Autodesk Inventor part; units mm, degrees
ref_plane "YZ Plane" through (0, 0, 0) normal (1, 0, 0) x (0, 1, 0)
ref_plane "XZ Plane" through (0, 0, 0) normal (0, 1, 0) x (-1, 0, 0)
ref_plane "XY Plane" through (0, 0, 0) normal (0, 0, 1) x (1, 0, 0)
sketch "스케치1" plane through (0, 0, 0) normal (1, 0, 0) x (0, 1, 0)
  line L0 (0, 0) -> (6, 0)
  line L1 (6, 0) -> (6, 15)
  line L2 (6, 15) -> (0, 15)
  line L3 (0, 15) -> (0, 0)
  line L4 (0, 15) -> (8, 15)
  line L5 (8, 15) -> (8, 40)
  line L6 (8, 40) -> (0, 40)
  line L7 (0, 40) -> (0, 15)
  line L8 (0, 40) -> (17, 40)
  line L9 (17, 40) -> (17, 55)
  line L10 (17, 55) -> (0, 55)
  line L11 (0, 55) -> (0, 40)
  line L12 (0, 55) -> (8, 55)
  line L13 (8, 55) -> (8, 80)
  line L14 (8, 80) -> (0, 80)
  line L15 (0, 80) -> (0, 55)
  line L16 (0, 80) -> (6, 80)
  line L17 (6, 80) -> (6, 120)
  line L18 (6, 120) -> (0, 120)
  line L19 (0, 120) -> (0, 80)
  dimension "d0" = 12
  dimension "d1" = 16
  dimension "d2" = 34
  dimension "d3" = 16
  dimension "d4" = 15
  dimension "d5" = 25
  dimension "d6" = 15
  dimension "d7" = 25
  dimension "d9" = 40
  dimension "d10" = 12
revolve "회전1" add sketch "스케치1" angle 360 about axis through (0, 0, 40) along (0, 0, -1)
sketch "스케치2" plane through (0, 0, 55) normal (0, 0, 1) x (1, 0, 0)
  circle A0 centre (0, 0) radius 8
  circle A1 centre (-4.5, 0) radius 12.5
  circle A2 centre (0, 0) radius 17
  point P0 (0, 0)
  dimension "d11" = 25
extrude "돌출1" cut sketch "스케치2" against normal up to next contours A2
sketch "스케치3" plane through (0, 0, 0) normal (0, 0, -1) x (-1, 0, 0)
  circle A0 centre (0, 0) radius 2
  dimension "d14" = 4
hole "구멍1" at (0, 0, 0) direction (0, 0, 1) diameter 3.242 depth 11.8 tip angle 118
sketch "스케치4" plane through (0, 0, 0) normal (1, 0, 0) x (0, 1, 0)
  line L0 (8, 78.2679) -> (8, 80)
  line L1 (8, 80) -> (7, 80)
  line L2 (7, 80) -> (8, 78.2679)
  line L3 (8, 80) -> (8, 55)
  line L4 (-8, 80) -> (8, 80)
  line L5 (0, -24) -> (0, 144)
  point P0 (0, 0)
  dimension "d22" = 30
  dimension "d23" = 1
revolve "회전2" cut sketch "스케치4" angle 360 about axis through (0, 0, -10) along (0, 0, 1)
fillet "모깎기1" radius 4 1 edges at (0, -8, 78.2679)
fillet "모깎기2" radius 1 1 edges at (0, -7, 80)
sketch "스케치5" plane through (0, 0, 0) normal (1, 0, 0) x (0, 1, 0)
  circle A0 centre (8.6, 98) radius 8
  line L0 (6, 120) -> (6, 80)
  point P0 (0, 0)
  dimension "d27" = 16
  dimension "d29" = 5.4
  dimension "d30" = 18
extrude "돌출2" cut sketch "스케치5" along normal mid plane 3
sketch "스케치6" plane through (0, 0, 0) normal (1, 0, 0) x (0, 1, 0)
  line L0 (-4.5, 105) -> (-6, 105)
  line L1 (-6, 105) -> (-6, 103.5)
  line L2 (-6, 103.5) -> (-4.5, 105)
  line L3 (-6, 120) -> (-6, 80)
  point P0 (0, 0)
  dimension "d33" = 1.5
  dimension "d34" = 45
  dimension "d35" = 25
revolve "회전3" cut sketch "스케치6" angle 360 about axis through (0, -4.5, 105) along (0, -1, 0)
chamfer "모따기1" distance 1 angle 45 3 edges at (0, -6, 120) (0, -8, 15) (0, -6, 0)
properties part number "3강"
For this review, take the finished solid that the model builds, in its own axes (mm). A direction names the side the tool comes from. Coordinates: 2 decimals unless noted, no trailing zeros. Order: outer loops, then holes, each group sorted by start corner. A loop starts at its lowest first (then second) coordinate and runs counter-clockwise, first axis right, second up. Notation, with made-up numbers: (45, 59) -> (77, 59) arc R11 ccw to (77, 65) -> close; hole circle Ø6 at (20, 33). An arc over 180 degrees is marked (long way). Use CSV: the item, a comma, the result in double quotes. Start each with the question number.
Item 1: Insertion check: pin 1 (5 mm diameter, centred on y = 3, z = 50, fed in from -X); pin 2 (6 mm diameter, centred on x = -4, z = 59.5, fed in from +Y); pin 3 (4 mm diameter, centred on y = -1, z = 37, fed in from -X). Each pin has a flat end and moves straight along its axis. Give the tip position at first contact, or say it passes through.
Item 2: We need section A-A, the plane z = 85.5. Give the boundary of the cut face in (x, y).
Item 3: Wall thickness on probe 1 along X at (y, z) = (0, 2.5); probe 2 along Z at (x, y) = (-15.75, 2.5); probe 3 along Y at (x, z) = (0.5, 83): over which ranges is each line inside the solid? List them lowest first.
Item 4: Draft analysis for pull direction X (two halves, no side actions). For faces 4 (the face through (0, 0.6, 98.1)), 5 (the face through (1.5, 4, 98)), 6 (the face through (2, 6, 15)), 7 (the face through (7.423, 3.755, 47.605)), state which applies: pulls with the +X half, pulls with the -X half, needs draft (parallel to the pull), parting line crosses it, or undercut.
Item 5: We need section B-B, the plane z = 70.5. Give the boundary of the cut face in (x, y), then the cut area to 3 significant figures.
Item 6: For faces 1 (the face through (0, -6, 8)), 2 (the face through (-1.802, 5.723, 99.773)), 3 (the face through (0, 0, 120)), list the 3-axis set-ups (+Z, -Z, +X, -X, +Y, -Y) from which the entire face can be reached by the end or side of a thin tool; tool diameter is ignored.
Derived:
1,pin 1,"stops at x = -16.99"
1,pin 2,"stops at y = 7.94"
1,pin 3,"stops at x = -8"
2,outline,"circle Ø12 at (0, 0)"
3,probe 1,"x = -6 to -1.62, 1.62 to 6"
3,probe 2,"z = 40 to 55"
3,probe 3,"y = -5.98 to 5.98"
4,face 4,"undercut"
4,face 5,"undercut"
4,face 6,"needs draft"
4,face 7,"parting line crosses it"
5,outline,"circle Ø16 at (0, 0)"
5,area,"201 mm^2"
6,face 1,"-Z"
6,face 2,"+Z"
6,face 3,"+Z, +X, -X, +Y, -Y"
